Study the drawing (mm; zero at the part's minimum x, y, z) and answer. A direction names the side the tool comes from. Round coordinates to 2 decimals unless told otherwise and drop trailing zeros. Write each loop counter-clockwise with the first axis right and the second up, starting at its lowest first coordinate (ties: lowest second). Pieces come first, ordered by that corner, then holes. Notation, with made-up numbers: M -33.75,16 L 20.25,16 A25 cw 20.25,47 Z; hole C 30.25,0 d10. An arc over 180 degrees is marked long. Put each result on its own line as item: value. Start each with the question number.
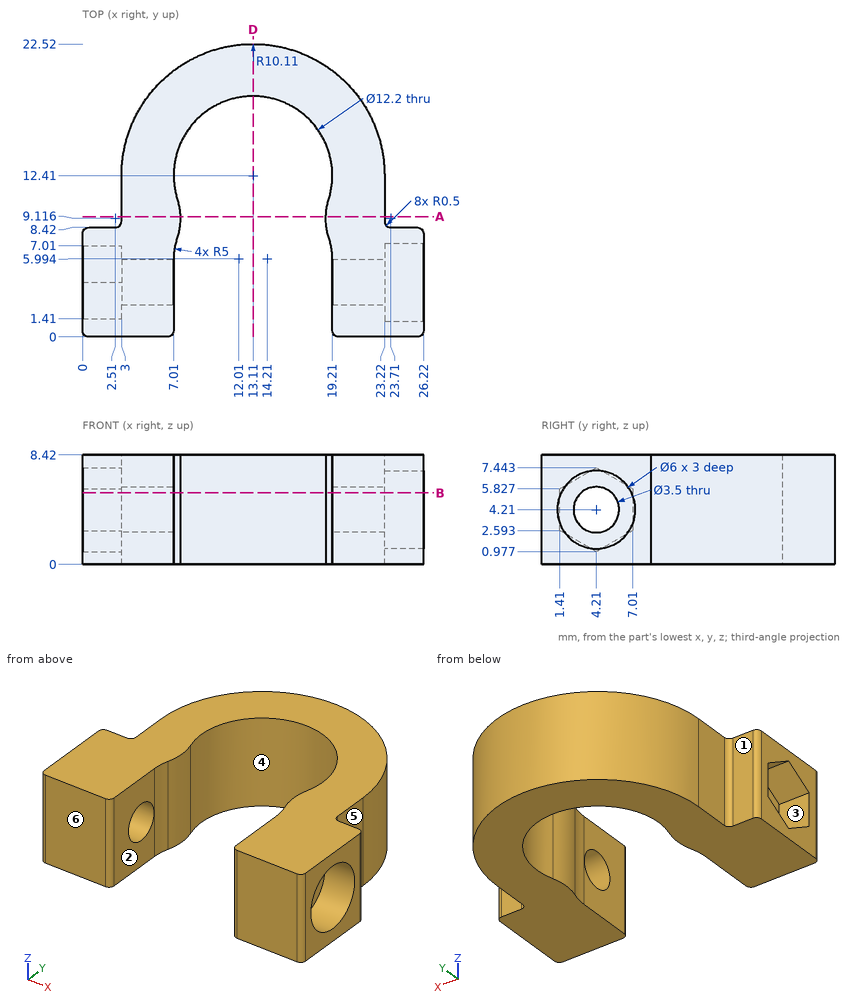
Item 1: Consider line 1 along X through (y, z) = (1.75, 3); line 2 along Y through (x, z) = (2, 5.75); line 3 along X through (y, z) = (5.25, 0.5). Determine where each line is inside the solid, lowest interval first. Write a range as [from, to].
Item 2: Which of the six approach directions +Z, -Z, +X, -X, +Y, -Y give full straight-line access (tool end or side, diameter ignored) to the marked faces 1, 2 and 3?
Item 3: Flat-ended cylindrical pins translate along their axes: pin 1 (1.6 mm diameter, centred on x = 2, z = 4, fed in from +Y); pin 2 (4 mm diameter, centred on y = 4.21, z = 4.21, fed in from -X); pin 3 (2 mm diameter, centred on x = 21.5, z = 3.5, fed in from +Y). Find the tip coordinate at first contact, or state that the pin passes through.
Item 4: Section D-D (x = 13.11) is taken. Give the vertices of the cut face in (y, z).
Item 5: Section B-B (z = 5.5) is taken. Count the separate pieces of the cut face and the enclosed holes in it, and give its area (3 significant figures).
Item 6: Section A-A (y = 9.25) is taken. Give the vertices of the cut face in (x, z).
Item 7: Determine the mould class of the marked faces 4, 5 and 6 for opening direction X: released by +X, released by -X, zero draft, split by the parting line, or undercut.
Output values:
1. line 1: x = [3, 7.01], [19.21, 23.22]
1. line 2: y = [0, 1.41], [7.01, 8.42]
1. line 3: x = [0, 7.01], [19.21, 26.22]
2. face 1: +Z, -Z, -X, +Y
2. face 2: +Z, -Z, -Y
2. face 3: -X
3. pin 1: stops at y = 8.52
3. pin 2: stops at x = 3
3. pin 3: stops at y = 19.31
4. outline: M 18.51,0 L 22.52,0 L 22.52,8.42 L 18.51,8.42 Z
5. separate pieces: 3
5. enclosed holes: 0
5. area: 203 mm^2
6. outline: M 3,0 L 7.51,0 L 7.51,8.42 L 3,8.42 Z; M 18.71,0 L 23.22,0 L 23.22,8.42 L 18.71,8.42 Z
7. face 4: undercut
7. face 5: released by +X
7. face 6: zero draft
